Here's how the part is built. I have some questions about the finished solid (model axes, mm). Face numbers are marked on the shaded views. A direction names the side the tool comes from. Give positions to 0.01 mm unless a question says otherwise; leave off trailing zeros. Loops run counter-clockwise (first coordinate to the right, second up) from the corner with the lowest first, then second, coordinate; pieces in that order, holes last. Notation, with made-up numbers: (51, -37.5) -> (102, -37.5) arc R24 cw to (102, -11.5) -> close; hole circle Ø2 at (-20.75, 18.25). An arc over 180 degrees is marked (long way). Answer in a Markdown table with one row per item. Add a question column.
Item 1: For P1, Ø12, axis at x = 2.5, y = 265, coming from the -Z side; P2, Ø12.5, axis at x = -18, z = 63, coming from the +Y side; P3, Ø2, axis at y = 230.5, z = 15, coming from the -X side; P4, Ø20.5, axis at x = -18.5, z = -23, coming from the -Y side, each with a flat end and sliding along its axis, tell me the tip position at first contact or that it passes through.
Item 2: Which directions (+Z, -Z, +X, -X, +Y, -Y) give clear straight access to the entire face, cutting with the end or side of a thin tool? Please do the marked faces 1, 2, 3 and 4.
Item 3: If we section it at A-A (z = 12.7): Write out the boundary of the cut face in (x, y).
Item 4: If we section it at B-B (y = 495.3): Write out the boundary of the cut face in (x, z), then the cut area to 3 significant figures.
Item 5: If we section it at C-C (z = 34.5): Write out the boundary of the cut face in (x, y), then the cut area to 3 significant figures.
Item 6: If we section it at D-D (x = -33): Write out the boundary of the cut face in (y, z), then the cut area to 3 significant figures.
Item 7: If I drill on line 1 (Y direction, x = -23, z = 57.5); line 2 (Z direction, x = -5, y = 393); line 3 (X direction, y = 277.5, z = 4.5), over which ranges is the centre line in solid material (lowest first)?
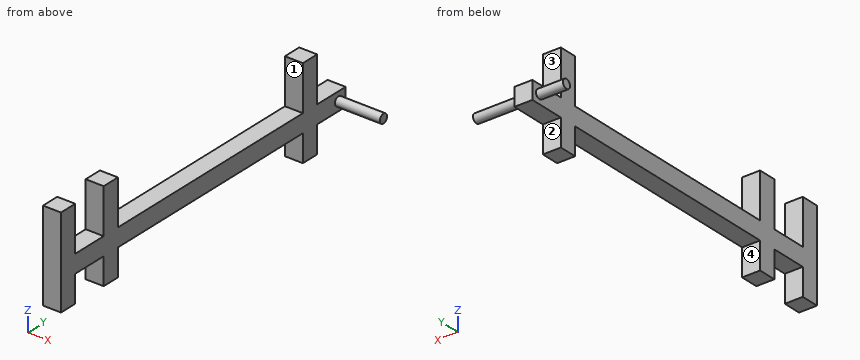
Autodesk Inventor part; units mm, degrees
ref_plane "YZ Plane" through (0, 0, 0) normal (1, 0, 0) x (0, 1, 0)
ref_plane "XZ Plane" through (0, 0, 0) normal (0, 1, 0) x (-1, 0, 0)
ref_plane "XY Plane" through (0, 0, 0) normal (0, 0, 1) x (1, 0, 0)
sketch "Sketch2" plane through (0, 0, 0) normal (0, 1, 0) x (-1, 0, 0)
  line L0 (0, 0) -> (25.4, 0)
  line L1 (25.4, 0) -> (25.4, 25.4)
  line L2 (25.4, 25.4) -> (0, 25.4)
  line L3 (0, 25.4) -> (0, 0)
  dimension "d0" = 25.4
  dimension "d1" = 25.4
extrude "Extrusion1" add sketch "Sketch2" along normal blind 508
sketch "Sketch3" plane through (0, 0, 25.4) normal (1, 0, 0) x (0, 0, -1)
  line L0 (25.4, 508) -> (0, 508)
  line L1 (25.4, 0) -> (25.4, 508)
  circle A0 centre (12.7, 495.3) radius 6.35
  dimension "d4" = 12.7
  dimension "d5" = 12.7
  dimension "d6" = 12.7
extrude "Extrusion2" add sketch "Sketch3" along normal mid plane 127
sketch "Sketch4" plane through (-25.4, 0, 25.4) normal (0, 0, 1) x (1, 0, 0)
  line L0 (25.4, 508) -> (0, 508)
  line L1 (0, 0) -> (0, 508)
  line L2 (0, 0) -> (25.4, 0)
  line L3 (25.4, 0) -> (25.4, 508)
  line L4 (0, 457.2) -> (25.4, 457.2)
  line L5 (25.4, 457.2) -> (25.4, 431.8)
  line L6 (25.4, 431.8) -> (0, 431.8)
  line L7 (0, 431.8) -> (0, 457.2)
  line L8 (0, 101.6) -> (25.4, 101.6)
  line L9 (25.4, 101.6) -> (25.4, 76.2)
  line L10 (25.4, 76.2) -> (0, 76.2)
  line L11 (0, 76.2) -> (0, 101.6)
  line L12 (0, 0) -> (25.4, 0)
  line L13 (25.4, 0) -> (25.4, 25.4)
  line L14 (25.4, 25.4) -> (0, 25.4)
  line L15 (0, 25.4) -> (0, 0)
  dimension "d9" = 25.4
  dimension "d10" = 50.8
  dimension "d11" = 25.4
  dimension "d13" = 330.2
  dimension "d14" = 381
  dimension "d17" = 25.4
  dimension "d18" = 101.6
extrude "Extrusion3" add sketch "Sketch4" along normal mid plane 127 contours L3 L6 L1 L4 | L3 L10 L1 L8 | L3 L2 L1 L14
properties part number "InnerTelescopeMockup"
Recorded:
| question | item | result |
|---|---|---|
| 1 | P1 | stops at z = 0 |
| 1 | P2 | stops at y = 457.2 |
| 1 | P3 | stops at x = -25.4 |
| 1 | P4 | stops at y = 0 |
| 2 | face 1 | +Z, +X, -X |
| 2 | face 2 | -Z, +X, -X, +Y |
| 2 | face 3 | +Z, +X, -X, +Y |
| 2 | face 4 | -Z, +X, -X |
| 3 | outline | (-63.5, 488.95) -> (-25.4, 488.95) -> (-25.4, 0) -> (0, 0) -> (0, 488.95) -> (63.5, 488.95) -> (63.5, 501.65) -> (0, 501.65) -> (0, 508) -> (-25.4, 508) -> (-25.4, 501.65) -> (-63.5, 501.65) -> close |
| 4 | outline | (-63.5, 6.35) -> (-25.4, 6.35) -> (-25.4, 0) -> (0, 0) -> (0, 6.35) -> (63.5, 6.35) -> (63.5, 19.05) -> (0, 19.05) -> (0, 25.4) -> (-25.4, 25.4) -> (-25.4, 19.05) -> (-63.5, 19.05) -> close |
| 4 | area | 1,940 mm^2 |
| 5 | outline | (-25.4, 0) -> (0, 0) -> (0, 25.4) -> (-25.4, 25.4) -> close; (-25.4, 76.2) -> (0, 76.2) -> (0, 101.6) -> (-25.4, 101.6) -> close; (-25.4, 431.8) -> (0, 431.8) -> (0, 457.2) -> (-25.4, 457.2) -> close |
| 5 | area | 1,940 mm^2 |
| 6 | outline | circle Ø12.7 at (495.3, 12.7) |
| 6 | area | 127 mm^2 |
| 7 | line 1 | y = 0 to 25.4, 76.2 to 101.6, 431.8 to 457.2 |
| 7 | line 2 | z = 0 to 25.4 |
| 7 | line 3 | x = -25.4 to 0 |
